Check sheet for the drawn part. Datum: minimum x, y, z corner. Units: mm. Give positions to 0.01 mm unless a question says otherwise; leave off trailing zeros. Order: outer loops, then holes, each group sorted by start corner. A loop starts at its lowest first (then second) coordinate and runs counter-clockwise, first axis right, second up. Notation, with made-up numbers: (32.25, 10) - (53.25, 10) arc R5 ccw to (53.25, 18) - close; hole circle Ø2 at (81, 69). An arc over 180 degrees is marked (long way). Answer as a JSON object with one key per item and string values. Group by question number.
(1) Section check A-A (z = 5). Record the boundary of the cut face in (x, y) (1 decimal).
(2) Section check D-D (x = 7.5). Record the boundary of the cut face in (y, z).
(3) Section check B-B (x = 5.25). Record the boundary of the cut face in (y, z).
(4) Section check C-C (y = 0.75). Record the boundary of the cut face in (x, z).
(5) Thickness scan on line 1 (X direction, y = 0.7, z = 4.5); line 2 (Z direction, x = 4.5, y = 0.4); line 3 (X direction, y = 0.2, z = 2.75) (1 decimal). Record the ranges inside material, lowest first.
(6) Depth check by flat-ended pin: pin 1 Ø4 at (x, z) = (4, 2.5) entering from -Y. Enter the tip coordinate at first touch or a pass-through.
(7) Mould release check, pull along X, two halves, no side actions. Record for the marked faces 1, 2 and 3: +X half, -X half, draft (parallel to the pull), parting line (faces both ways), or undercut.
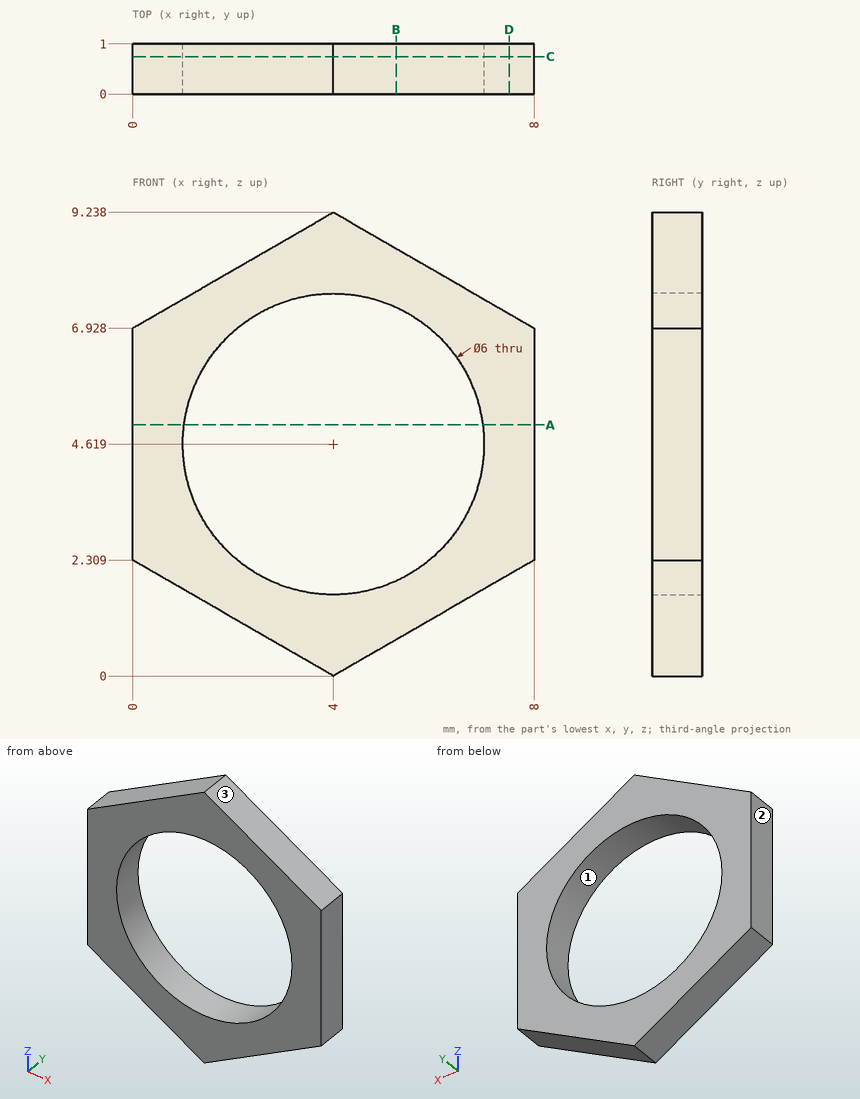
Solutions:
{
 "1": {"outline": "(0, 0) - (1, 0) - (1, 1) - (0, 1) - close; (7, 0) - (8, 0) - (8, 1) - (7, 1) - close"},
 "2": {"outline": "(0, 2.02) - (1, 2.02) - (1, 7.22) - (0, 7.22) - close"},
 "3": {"outline": "(0, 0.72) - (1, 0.72) - (1, 1.89) - (0, 1.89) - close; (0, 7.35) - (1, 7.35) - (1, 8.52) - (0, 8.52) - close"},
 "4": {"outline": "(0, 2.31) - (4, 0) - (8, 2.31) - (8, 6.93) - (4, 9.24) - (0, 6.93) - close; hole circle Ø6 at (4, 4.62)"},
 "5": {"line 1": "x = 0 to 1, 7 to 8", "line 2": "z = 0.29 to 1.66, 7.58 to 8.95", "line 3": "x = 0 to 1.7, 6.3 to 8"},
 "6": {"pin 1": "stops at y = 0"},
 "7": {"face 1": "undercut", "face 2": "-X half", "face 3": "+X half"}
}
